```python
from build123d import *

# Parameters (mm, degrees)
F0_R     = 1.75
F0_W     = 17
F0_H     = 9.7
F1_DEPTH = 6.35
F0_R_2   = 4.5
F2_DEPTH = 3.175


# Not quite as in the source:
# - a length typed as a fraction of an inch, garbled in the dataset ("3 / 203.2 mm" for 3/8 in), is restored


with BuildPart() as f1:
    # F0 (on Top) → F1 (new body)
    with BuildSketch(Plane.XY):
        Polygon((9.9961940777, 6.35), (-9.9961940777, 6.35), (-15, 1.3461940777), (-15, -1.3461940777), (-9.9961940777, -6.35), (9.9961940777, -6.35), (15, -1.3461940777), (15, 1.3461940777), align=None)
        with Locations((-11.75, 0)):
            Circle(F0_R, mode=Mode.SUBTRACT)
        Rectangle(F0_W, F0_H, mode=Mode.SUBTRACT)
        with Locations((11.75, 0)):
            Circle(F0_R, mode=Mode.SUBTRACT)
    extrude(amount=F1_DEPTH)

    # F0 (on Top) → F2 (join)
    with BuildSketch(Plane.XY):
        Rectangle(F0_W, F0_H)
        Circle(F0_R_2, mode=Mode.SUBTRACT)
    extrude(amount=F2_DEPTH)


solid = f1.part
```
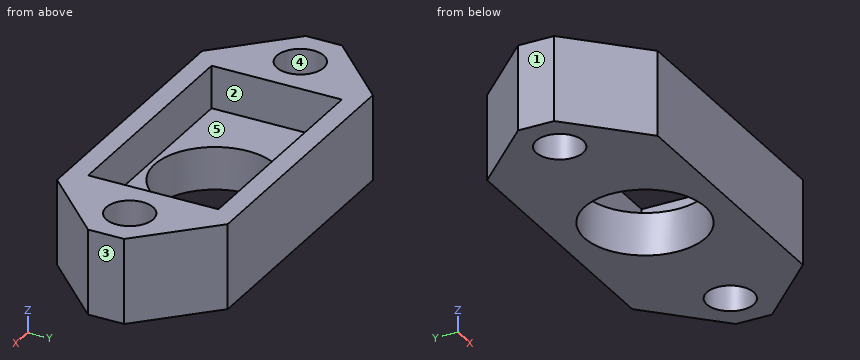
The listing builds one solid part. Answer for the finished solid, in the listing's coordinates (mm). Face numbers are marked on the shaded views. A direction names the side the tool comes from. Give positions to 0.01 mm unless a question says otherwise; leave off trailing zeros. Order: outer loops, then holes, each group sorted by start corner. A loop starts at its lowest first (then second) coordinate and runs counter-clockwise, first axis right, second up.
1) Determine the mould class of the marked faces 1, 2 and 3 for opening direction X: pulls with the +X half, pulls with the -X half, needs draft (parallel to the pull), parting line crosses it, or undercut.
Reported:
face 1: pulls with the -X half
face 2: undercut
face 3: pulls with the +X half
2) For the marked faces 4 and 5, determine the directions among +Z, -Z, +X, -X, +Y, -Y from which every point of the face is accessible in a straight line to the end or side of a thin tool.
Reported:
face 4: +Z, -Z
face 5: +Z
3) Find section D-D on y = 3.75. Write down the section's boundary in (x, z) (3 decimals), then the cut area to 3 significant figures.
Reported:
outline: (-12.596, 0) - (-2.487, 0) - (-2.487, 3.175) - (-8.5, 3.175) - (-8.5, 6.35) - (-12.596, 6.35) - close; (2.487, 0) - (12.596, 0) - (12.596, 6.35) - (8.5, 6.35) - (8.5, 3.175) - (2.487, 3.175) - close
area: 90.2 mm2
4) Find section C-C on y = 0. Write down the section's boundary in (x, z) (3 decimals).
Reported:
outline: (-15, 0) - (-13.5, 0) - (-13.5, 6.35) - (-15, 6.35) - close; (-10, 0) - (-4.5, 0) - (-4.5, 3.175) - (-8.5, 3.175) - (-8.5, 6.35) - (-10, 6.35) - close; (4.5, 0) - (10, 0) - (10, 6.35) - (8.5, 6.35) - (8.5, 3.175) - (4.5, 3.175) - close; (13.5, 0) - (15, 0) - (15, 6.35) - (13.5, 6.35) - close
5) Given P1, Ø3, axis at y = 4, z = 2, coming from the +X side; P2, Ø1, axis at y = 2.5, z = 2.5, coming from the +X side; P3, Ø1.5, axis at x = 11, z = 3.5, coming from the -Y side, each flat-ended and moving along its own axis, determine where each tip first touches the part or whether it passes through.
Reported:
P1: stops at x = 13.85
P2: stops at x = 14.35
P3: stops at y = -6.1
6) Find section B-B on z = 4.25. Write down the section's boundary in (x, y).
Reported:
outline: (-15, -1.35) - (-10, -6.35) - (10, -6.35) - (15, -1.35) - (15, 1.35) - (10, 6.35) - (-10, 6.35) - (-15, 1.35) - close; hole circle Ø3.5 at (-11.75, 0); hole (-8.5, -4.85) - (8.5, -4.85) - (8.5, 4.85) - (-8.5, 4.85) - close; hole circle Ø3.5 at (11.75, 0)
7) Find section A-A on x = 0. Write down the section's boundary in (y, z) (3 decimals).
Reported:
outline: (-6.35, 0) - (-4.5, 0) - (-4.5, 3.175) - (-4.85, 3.175) - (-4.85, 6.35) - (-6.35, 6.35) - close; (4.5, 0) - (6.35, 0) - (6.35, 6.35) - (4.85, 6.35) - (4.85, 3.175) - (4.5, 3.175) - close
8) Consider line 1 along Y through (x, z) = (-5.5, 3.5); line 2 along Y through (x, z) = (0, 1.15); line 3 along X through (y, z) = (-0.5, 5.5). Determine where each line is inside the solid, lowest interval first.
Reported:
line 1: y = -6.35 to -4.85, 4.85 to 6.35
line 2: y = -6.35 to -4.5, 4.5 to 6.35
line 3: x = -15 to -13.43, -10.07 to -8.5, 8.5 to 10.07, 13.43 to 15
